Autodesk Fusion 360 part; units mm, degrees
sketch "Sketch1" plane through (0, 0, 0) normal (1, 0, 0) x (0, 1, 0)
  line L0 (0, 0) -> (0, 6.5)
  line L1 (0, 6.5) -> (13, 9.9833)
  line L2 (0, 6.5) -> (200, 6.5) construction
  line L3 (0, 0) -> (0, 6.5)
  line L4 (0, 10) -> (13, 10)
  line L5 (13, 10) -> (13, 6.5)
  line L6 (-2, 6.5) -> (0, 6.5)
  line L7 (-2, 0) -> (0, 0)
  line L8 (-2, 6.5) -> (-28.4207, 25)
  line L9 (-2, 6.5) -> (198, 6.5) construction
  line L10 (0, 25) -> (-28.4207, 25)
  line L11 (0, 0) -> (0, 6.5)
  line L12 (0, 10) -> (0, 25)
  line L13 (13, 9.9833) -> (13, 25)
  line L14 (13, 25) -> (0, 25)
  line L15 (-28.4207, 25) -> (-18.4207, 25)
  line L16 (-18.4207, 25) -> (-16.4207, 25)
  line L17 (-16.4207, 25) -> (-16.4207, 24)
  line L18 (-16.4207, 24) -> (-18.4207, 24)
  line L19 (-18.4207, 24) -> (-18.4207, 25)
  line L20 (-16.4207, 25) -> (-6.4207, 25)
  line L21 (-6.4207, 25) -> (-4.4207, 25)
  line L22 (-4.4207, 25) -> (-4.4207, 24)
  line L23 (-4.4207, 24) -> (-6.4207, 24)
  line L24 (-6.4207, 24) -> (-6.4207, 25)
  dimension "d7" = 6.5
  dimension "d8" = 15
  dimension "d10" = 10
  dimension "d11" = 6.5
  dimension "d12" = 145
  dimension "d14" = 25
  dimension "d15" = 10
  dimension "d16" = 2
  dimension "d17" = 1
  dimension "d18" = 10
  dimension "d19" = 2
  dimension "d20" = 1
revolve "Revolve1" add sketch "Sketch1" angle 360 about axis through (0, 1.75, 0) along (0, 1, 0) contours L1 L4 L5 L6 L8 L10 L12 L13 L15 L17 L18 L19 L20 L22 L23 L24 | L4 L12 L13 L14
Model file for the job. Use its own axes, mm. A direction names the side the tool comes from. Give positions to 0.01 mm unless a question says otherwise; leave off trailing zeros. Order: outer loops, then holes, each group sorted by start corner. A loop starts at its lowest first (then second) coordinate and runs counter-clockwise, first axis right, second up. Notation, with made-up numbers: (68.25, 32.5) - (124.25, 32.5) arc R31 cw to (124.25, 67.5) - close; hole circle Ø4 at (46.5, -37.5). An arc over 180 degrees is marked (long way). One line per item, written item: value.
Item 1: Slice it at B-B (z = 0). List the corners of the cut face in (x, y), then the cut area to 4 significant figures.
Response values:
outline: (-25, -28.42) - (-6.5, -2) - (-6.5, 0) - (-9.98, 13) - (-25, 13) - (-25, -4.42) - (-24, -4.42) - (-24, -6.42) - (-25, -6.42) - (-25, -16.42) - (-24, -16.42) - (-24, -18.42) - (-25, -18.42) - close; (6.5, -2) - (25, -28.42) - (25, -18.42) - (24, -18.42) - (24, -16.42) - (25, -16.42) - (25, -6.42) - (24, -6.42) - (24, -4.42) - (25, -4.42) - (25, 13) - (9.98, 13) - (6.5, 0) - close
area: 990.5 mm2
Item 2: Tool access for faces 1 (the cylindrical face through (-1.055, -17.435, -23.977)), 2 (the flat face through (-11, 13, 0)): list every direction of +Z, -Z, +X, -X, +Y, -Y with a clear straight run to the whole face (end or side of a thin tool).
Response values:
face 1: none
face 2: +Z, -Z, +X, -X, +Y
Item 3: Slice it at C-C (y = 8.5). List the corners of the cut face in (x, z), then the cut area to 3 significant figures.
Response values:
outline: circle Ø50 at (0, 0); hole circle Ø17.56 at (0, 0)
area: 1,720 mm2
Item 4: Two-plate mould, pull along Z, no slides. Class faces 3 (the cylindrical face through (-3.955, -0.986, -5.158)), 4 (the flat face through (22.3, -18.421, -9.4)), 5 (the cylindrical face through (-7.509, -11.491, 23.846)): released by +Z, released by -Z, zero draft, split by the parting line, or undercut.
Response values:
face 3: undercut
face 4: zero draft
face 5: split by the parting line
Item 5: Slice it at A-A (x = 0). List the corners of the cut face in (y, z).
Response values:
outline: (-28.42, -25) - (-18.42, -25) - (-18.42, -24) - (-16.42, -24) - (-16.42, -25) - (-6.42, -25) - (-6.42, -24) - (-4.42, -24) - (-4.42, -25) - (13, -25) - (13, -9.98) - (0, -6.5) - (-2, -6.5) - close; (-28.42, 25) - (-2, 6.5) - (0, 6.5) - (13, 9.98) - (13, 25) - (-4.42, 25) - (-4.42, 24) - (-6.42, 24) - (-6.42, 25) - (-16.42, 25) - (-16.42, 24) - (-18.42, 24) - (-18.42, 25) - close
Item 6: Slice it at D-D (y = -9). List the corners of the cut face in (x, z).
Response values:
outline: circle Ø50 at (0, 0); hole circle Ø22.8 at (0, 0)
Item 7: Wall check: line 1 (X direction, y = -1.15, z = 0); line 2 (Y direction, x = -21.5, z = -12.5); line 3 (X direction, y = -13, z = -9.5). Give the ranges that are in metal, low to high.
Response values:
line 1: -25 to -6.5, 6.5 to 25
line 2: -28.23 to -18.42, -16.42 to -6.42, -4.42 to 13
line 3: -23.12 to -10.56, 10.56 to 23.12
Item 8: Pin check, flat tips, straight feed: pin 1 Ø4 at (y, z) = (-4.5, -0.5) entering from +X; pin 2 Ø15 at (x, z) = (11.5, 10.5) entering from -Y; pin 3 Ø2 at (x, y) = (16, -8) entering from -Z. Stop position of each tip, or through.
Response values:
pin 1: x = 25
pin 2: y = -25.67
pin 3: z = -20
